Autodesk Inventor part; units mm, degrees
ref_plane "YZ Plane" through (0, 0, 0) normal (1, 0, 0) x (0, 1, 0)
ref_plane "XZ Plane" through (0, 0, 0) normal (0, 1, 0) x (-1, 0, 0)
ref_plane "XY Plane" through (0, 0, 0) normal (0, 0, 1) x (1, 0, 0)
sketch "Sketch1" plane through (0, 0, 0) normal (0, 1, 0) x (-1, 0, 0)
  circle A0 centre (0, 0) radius 11.1
  circle A1 centre (0, 0) radius 20.1
  circle A2 centre (0, 15.6) radius 2.5
  circle A3 centre (0, 0) radius 9.1
  dimension "d0" = 22.2
  dimension "d1" = 9
  dimension "d3" = 5
  dimension "d4" = 15.6
  dimension "d9" = 2
  dimension "d17" = 18.2
extrude "Extrusion1" add sketch "Sketch1" along normal blind 7 contours A1 | A2
extrude "Extrusion3" add sketch "Sketch1" against normal blind 3 contours A0 | A1 | A2
extrude "Extrusion4" cut sketch "Sketch1" along normal through all both and the other way through all contours A2
pattern_circular "Circular Pattern1" count 6 over 360 about axis through (0, 0, 0) along (0, -1, 0) of "Extrusion4"
equation "\"d4\" = 0.5 * d1 + 0.5 * d0"
properties part number "Csapagyhaz"
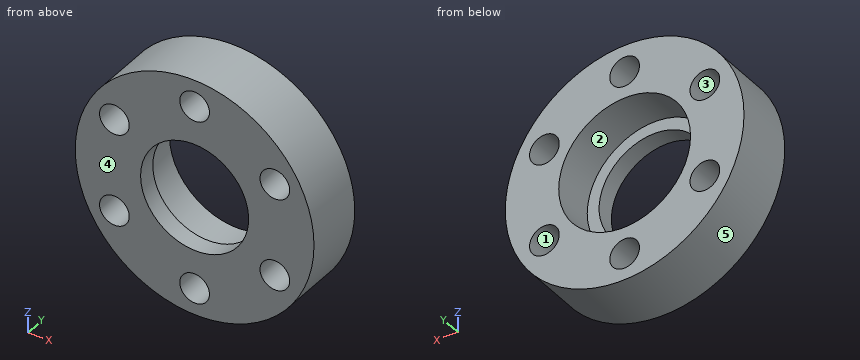
Part model, mm, in its own coordinate system. Face numbers are marked on the shaded views. A direction names the side the tool comes from. Coordinates: 2 decimals unless noted, no trailing zeros. Loops run counter-clockwise (first coordinate to the right, second up) from the corner with the lowest first, then second, coordinate; pieces in that order, holes last. Notation, with made-up numbers: (46.5, 21.5) -> (78.5, 21.5) arc R10 cw to (78.5, 30.5) -> close; hole circle Ø4 at (-35.75, -12). An arc over 180 degrees is marked (long way). Use a Markdown table: item, result. Add a question column.
Item 1: Pull direction X, two halves, no side cores. Call the marked faces 3, 4 and 5: +X half, -X half, draft (parallel to the pull), parting line (faces both ways), or undercut.
Item 2: Band-saw the part on D-D on y = -0.75. Write the cut outline in (x, z).
Item 3: Band-saw the part on A-A on z = 0. Write the cut outline in (x, y), plus the area to 3 significant figures.
Item 4: Band-saw the part on B-B on z = -7.8. Write the cut outline in (x, y), plus the area to 3 significant figures.
Item 5: Which spindle directions (+Z, -Z, +X, -X, +Y, -Y) get a long thin tool onto all of the face, cutting with end or side? Do the marked faces 1 and 2. Say none if no direction does.
Item 6: Band-saw the part on C-C on x = -0.5. Write the cut outline in (y, z).
Item 7: Flat gauge pins, fed straight in: P1, Ø4.5, axis at x = 13.51, z = 7.8, coming from the +Y side; P2, Ø4, axis at x = 14.5, z = 7.5, coming from the +Y side; P3, Ø1.5, axis at y = 0.5, z = 8.5, coming from the +X side; P4, Ø2, axis at y = 5, z = 3.5, coming from the -X side. Where does each tip first touch, or does it go through?
Item 8: Probe probe 1 along X at (y, z) = (3.25, -8.5); probe 2 along Z at (x, y) = (-1, -1.5); probe 3 along Z at (x, y) = (-14, 1). List the from-to ranges inside material, lowest first.
Geometry says:
| question | item | result |
|---|---|---|
| 1 | face 3 | undercut |
| 1 | face 4 | draft |
| 1 | face 5 | parting line |
| 2 | outline | circle Ø40.2 at (0, 0); hole circle Ø5 at (-13.51, -7.8); hole circle Ø5 at (-13.51, 7.8); hole circle Ø18.2 at (0, 0); hole circle Ø5 at (0, -15.6); hole circle Ø5 at (0, 15.6); hole circle Ø5 at (13.51, -7.8); hole circle Ø5 at (13.51, 7.8) |
| 3 | outline | (-20.1, -3) -> (-9.1, -3) -> (-9.1, 0) -> (-11.1, 0) -> (-11.1, 7) -> (-20.1, 7) -> close; (9.1, -3) -> (20.1, -3) -> (20.1, 7) -> (11.1, 7) -> (11.1, 0) -> (9.1, 0) -> close |
| 3 | area | 192 mm² |
| 4 | outline | (-18.52, -3) -> (-16.01, -3) -> (-16.01, 7) -> (-18.52, 7) -> close; (-11.01, -3) -> (-4.69, -3) -> (-4.69, 0) -> (-7.9, 0) -> (-7.9, 7) -> (-11.01, 7) -> close; (4.69, -3) -> (11.01, -3) -> (11.01, 7) -> (7.9, 7) -> (7.9, 0) -> (4.69, 0) -> close; (16.01, -3) -> (18.52, -3) -> (18.52, 7) -> (16.01, 7) -> close |
| 4 | area | 132 mm² |
| 5 | face 1 | +Y, -Y |
| 5 | face 2 | +Y |
| 6 | outline | (-3, -20.09) -> (7, -20.09) -> (7, -18.05) -> (-3, -18.05) -> close; (-3, -13.15) -> (7, -13.15) -> (7, -11.09) -> (0, -11.09) -> (0, -9.09) -> (-3, -9.09) -> close; (-3, 9.09) -> (0, 9.09) -> (0, 11.09) -> (7, 11.09) -> (7, 13.15) -> (-3, 13.15) -> close; (-3, 18.05) -> (7, 18.05) -> (7, 20.09) -> (-3, 20.09) -> close |
| 7 | P1 | through |
| 7 | P2 | y = 7 |
| 7 | P3 | x = 18.55 |
| 7 | P4 | x = -19.94 |
| 8 | probe 1 | -18.21 to -15.91, -11.11 to -7.14, 7.14 to 11.11, 15.91 to 18.21 |
| 8 | probe 2 | -20.08 to -17.89, -13.31 to -9.04, 9.04 to 13.31, 17.89 to 20.08 |
| 8 | probe 3 | -14.42 to -10.25, -5.35 to 5.35, 10.25 to 14.42 |
